from build123d import *

# Parameters (mm, degrees)
SKETCH2_W             = 9.5
SKETCH2_H             = 9.5
SKETCH2_R             = 2.65
BOSS_EXTRUDE1_DEPTH   = 10
BOSS_EXTRUDE1_2_DEPTH = 10
SKETCH13_W            = 49.5
SKETCH13_H            = 50
BOSS_EXTRUDE4_DEPTH   = 2
CUT_EXTRUDE3_START    = 2
SKETCH12_R            = 1.6
CUT_EXTRUDE3_DEPTH    = 2
SKETCH14_R            = 3
BOSS_EXTRUDE5_DEPTH   = 5
SKETCH15_W            = 9.5
SKETCH15_H            = 4
BOSS_EXTRUDE6_DEPTH   = 2


with BuildPart() as part:
    # Sketch2 → Boss-Extrude1 (new body)
    with BuildSketch(Plane(origin=(0, 0, 0), x_dir=(1, 0, 0), z_dir=(0, 1, 0))):
        with Locations((4.75, 4.75)):
            Rectangle(SKETCH2_W, SKETCH2_H)
        with Locations((4.75, 4.75)):
            Circle(SKETCH2_R, mode=Mode.SUBTRACT)
    extrude(amount=BOSS_EXTRUDE1_DEPTH)



with BuildPart() as body_2:
    # Sketch2 → Boss-Extrude1 2 (new body)
    with BuildSketch(Plane(origin=(0, 0, 0), x_dir=(1, 0, 0), z_dir=(0, 1, 0))):
        with Locations((44.75, 4.75)):
            Rectangle(SKETCH2_W, SKETCH2_H)
        with Locations((44.75, 4.75)):
            Circle(SKETCH2_R, mode=Mode.SUBTRACT)
    extrude(amount=BOSS_EXTRUDE1_2_DEPTH)


with BuildPart() as part_1:
    add(part.part)

    add(body_2.part)  # Boss-Extrude4 merges body 2
    # Sketch13 → Boss-Extrude4 (add)
    with BuildSketch(Plane.XY):
        with Locations((24.75, 29)):
            Rectangle(SKETCH13_W, SKETCH13_H)
    extrude(amount=BOSS_EXTRUDE4_DEPTH)

    # Sketch12 → Cut-Extrude3 (cut)
    with BuildSketch(Plane.XY.offset(CUT_EXTRUDE3_START)):
        with Locations((24.75, 8.1)):
            Circle(SKETCH12_R)
        with Locations((8.81513257, 35.7)):
            Circle(SKETCH12_R)
        with Locations((40.68486743, 35.7)):
            Circle(SKETCH12_R)
    extrude(amount=-CUT_EXTRUDE3_DEPTH, mode=Mode.SUBTRACT)

    # Sketch14 → Boss-Extrude5 (add)
    with BuildSketch(Plane(origin=(0, 0, 0), x_dir=(-1, 0, 0), z_dir=(0, 0, -1))):
        with BuildLine():
            Line((-9.5, 54), (-40, 54))
            Line((-40, 54), (-40, 38.620780136))
            ThreePointArc((-40, 38.620780136), (-38.333846131, 37.563517871), (-37.68486743, 35.7))
            ThreePointArc((-37.68486743, 35.7), (-38.333846131, 33.836482129), (-40, 32.779219864))
            Line((-40, 32.779219864), (-40, 10))
            Line((-40, 10), (-40, 4))
            Line((-40, 4), (-9.5, 4))
            Line((-9.5, 4), (-9.5, 10))
            Line((-9.5, 10), (-9.5, 32.779219864))
            ThreePointArc((-9.5, 32.779219864), (-11.81513257, 35.7), (-9.5, 38.620780136))
            Line((-9.5, 38.620780136), (-9.5, 54))
        make_face()
        with Locations((-24.75, 8.1)):
            Circle(SKETCH14_R, mode=Mode.SUBTRACT)
    extrude(amount=BOSS_EXTRUDE5_DEPTH)

    # Sketch15 → Boss-Extrude6 (add)
    with BuildSketch(Plane.XY):
        with Locations((4.75, 2)):
            Rectangle(SKETCH15_W, SKETCH15_H)
        with Locations((44.75, 2)):
            Rectangle(SKETCH15_W, SKETCH15_H)
    extrude(amount=BOSS_EXTRUDE6_DEPTH)


solid = part_1.part
Could you check a few things on this model? Use its own coordinates, in mm. A direction names the side the tool comes from. Coordinates: 2 decimals unless noted, no trailing zeros. Loops run counter-clockwise (first coordinate to the right, second up) from the corner with the lowest first, then second, coordinate; pieces in that order, holes last.
1. Imagine slicing it at C-C (z = -3.75). Please give me the cut outline in (x, y).
2. Imagine slicing it at B-B (x = 4.75). Please give me the cut outline in (y, z), and give its area (3 significant figures).
3. For P1, Ø5, axis at x = 44.75, z = -4.75, coming from the -Y side (3 decimals); P2, Ø5, axis at x = 26, y = 8.5, coming from the -Z side; P3, Ø6, axis at x = 46.5, y = 29.5, coming from the -Z side; P4, Ø2, axis at x = 32, z = -1.5, coming from the -Y side, each with a flat end and sliding along its axis, tell me the tip position at first contact or that it passes through.
4. I need wall thicknesses on L1, parallel to Z at x = 4.75, y = 7.25; L2, parallel to X at y = 4, z = -8.25; L3, parallel to Y at x = 24.75, z = 0.6. Which ranges of each line are inside material? Lowest first, please.
5. For faces 5 (the face through (25.141, 11.074, -2.465)), 6 (the face through (9.5, 3.8, -5.1)), 7 (the face through (9.5, 21, -2)), 8 (the face through (24, 27, 2)), 9 (the face through (40, 46, -2)), which set-ups out of +Z, -Z, +X, -X, +Y, -Y let a thin tool reach every point of the face, with its end or its side?
6. We'd pull the mould along X, two halves only. Please class faces 1 (the face through (40, 22, -2)), 2 (the face through (7.2, 4.93, -3.74)), 3 (the face through (40, 3.8, -5.1)), 4 (the face through (11.815, 35.644, -2.465)): released by +X, released by -X, zero draft, split by the parting line, or undercut.
7. Imagine slicing it at D-D (x = 24.75). Please give me the cut outline in (y, z).
8. Imagine slicing it at A-A (y = 8.1). Please give me the cut outline in (x, z).
Computed values:
1. outline: (0, 0) - (2.3, 0) - (2.3, 10) - (0, 10) - close; (7.2, 0) - (9.5, 0) - (9.5, 4) - (40, 4) - (40, 0) - (42.3, 0) - (42.3, 10) - (40, 10) - (40, 32.78) arc R3 cw to (40, 38.62) - (40, 54) - (9.5, 54) - (9.5, 38.62) arc R3 cw to (9.5, 32.78) - (9.5, 10) - (7.2, 10) - close; (47.2, 0) - (49.5, 0) - (49.5, 10) - (47.2, 10) - close; hole circle Ø6 at (24.75, 8.1)
2. outline: (0, -9.5) - (10, -9.5) - (10, -7.4) - (0, -7.4) - close; (0, -2.1) - (10, -2.1) - (10, 0) - (54, 0) - (54, 2) - (0, 2) - close
2. area: 150 mm2
3. P1: passes through
3. P2: stops at z = -5
3. P3: stops at z = 0
3. P4: stops at y = 4
4. L1: z = -9.5 to -7.4, -2.1 to 2
4. L2: x = 0 to 9.5, 40 to 49.5
4. L3: y = 4 to 6.5, 9.7 to 54
5. face 5: -Z
5. face 6: -Z, -Y
5. face 7: -Z, -X, +Y
5. face 8: +Z, +X, -X, +Y, -Y
5. face 9: -Z, +X, +Y
6. face 1: released by +X
6. face 2: undercut
6. face 3: undercut
6. face 4: released by -X
7. outline: (4, -5) - (5.1, -5) - (5.1, 0) - (6.5, 0) - (6.5, 2) - (4, 2) - close; (9.7, 0) - (11.1, 0) - (11.1, -5) - (54, -5) - (54, 2) - (9.7, 2) - close
8. outline: (0, -9.5) - (9.5, -9.5) - (9.5, -5) - (21.75, -5) - (21.75, 0) - (23.15, 0) - (23.15, 2) - (0, 2) - close; (26.35, 0) - (27.75, 0) - (27.75, -5) - (40, -5) - (40, -9.5) - (49.5, -9.5) - (49.5, 2) - (26.35, 2) - close; hole circle Ø5.3 at (4.75, -4.75); hole circle Ø5.3 at (44.75, -4.75)
